```python
from build123d import *

# Parameters (mm, degrees)
SKETCH_1_W          = 8
SKETCH_1_H          = 8
EXTRUDE_1_DEPTH     = 35
SKETCH_2_R          = 1.65
CUT_EXTRUDE_1_DEPTH = 40
SKETCH_3_R          = 1.65
CUT_EXTRUDE_2_DEPTH = 40
SKETCH_6_R          = 1.5
CUT_EXTRUDE_4_DEPTH = 37.783148315
HOLE_WIZARD_M4_3_D  = 3.3


with BuildPart() as part:
    # 草图1 → 凸台-拉伸1 (new body)
    with BuildSketch(Plane.XY):
        with Locations((4, 4)):
            Rectangle(SKETCH_1_W, SKETCH_1_H)
    extrude(amount=EXTRUDE_1_DEPTH)

    # 草图2 → 切除-拉伸1 (cut)
    with BuildSketch(Plane(origin=(8, 0, 0), x_dir=(0, 0, -1), z_dir=(1, 0, 0))):
        with Locations(Location((-32.5, 4, 0), (0, 0, 90))):
            Circle(SKETCH_2_R)
        with Locations(Location((-2.5, 4, 0), (0, 0, 90))):
            Circle(SKETCH_2_R)
    extrude(amount=-CUT_EXTRUDE_1_DEPTH, mode=Mode.SUBTRACT)

    # 草图3 → 切除-拉伸2 (cut)
    with BuildSketch(Plane(origin=(0, 8, 0), x_dir=(1, 0, 0), z_dir=(0, 1, 0))):
        with Locations(Location((4, -17.5, 0), (0, 0, 270))):
            Circle(SKETCH_3_R)
    extrude(amount=-CUT_EXTRUDE_2_DEPTH, mode=Mode.SUBTRACT)

    # 草图6 → 切除-拉伸4 (cut, through all)
    with BuildSketch(Plane(origin=(8, 0, 0), x_dir=(0, 0, -1), z_dir=(1, 0, 0))):
        with Locations(Location((-17.5, 4, 0), (0, 0, 90))):
            Circle(SKETCH_6_R)
    extrude(amount=-CUT_EXTRUDE_4_DEPTH, mode=Mode.SUBTRACT)

    # M4 螺纹孔3 (through all)
    with Locations(Plane(origin=(8, 0, 0), x_dir=(0, 0, -1), z_dir=(1, 0, 0))):
        with Locations((-17.5, 4)):
            Hole(HOLE_WIZARD_M4_3_D / 2)


solid = part.part
```
Input: part model. Units: mm. Frame: model coordinates. Give positions to 0.01 mm unless a question says otherwise; leave off trailing zeros. Order: outer loops, then holes, each group sorted by start corner. A loop starts at its lowest first (then second) coordinate and runs counter-clockwise, first axis right, second up. Notation, with made-up numbers: (72, 11.25) - (120, 11.25) arc R18 ccw to (120, 26.25) - close; hole circle Ø9 at (69, 38.25). An arc over 180 degrees is marked (long way). One line per item, written item: value.
1. Cut plane B-B, the plane z = 32.5. Output: boundary loops of the cut face in (x, y), and give its area (3 significant figures).
Determined:
outline: (0, 0) - (8, 0) - (8, 2.35) - (0, 2.35) - close; (0, 5.65) - (8, 5.65) - (8, 8) - (0, 8) - close
area: 37.6 mm2
2. Line query: probe 1 along Z at (x, y) = (4.5, 4); probe 2 along X at (y, z) = (5.7, 17.5); probe 3 along Z at (x, y) = (2, 5). Output: solid intervals per line, ascending.
Determined:
probe 1: 0 to 0.85, 4.15 to 15.85, 19.15 to 30.85, 34.15 to 35
probe 2: 0 to 2.35, 5.65 to 8
probe 3: 0 to 1.19, 3.81 to 16.19, 18.81 to 31.19, 33.81 to 35
3. Cut plane C-C, the plane y = 6.75. Output: boundary loops of the cut face in (x, z).
Determined:
outline: (0, 0) - (8, 0) - (8, 35) - (0, 35) - close; hole circle Ø3.3 at (4, 17.5)
4. Draft query along Z for faces 1 (the face through (6, 8, 17)), 2 (the face through (1.53, 4.07, 15.85)), 3 (the face through (4, 4, 0)). Return one class per face: released by +Z, released by -Z, zero draft, split by the parting line, or undercut.
Determined:
face 1: zero draft
face 2: undercut
face 3: released by -Z
5. Pin query (flat end, axial travel): pin 1 Ø3 at (y, z) = (4, 17.5) entering from +X. Return the tip coordinate at first contact, or that it passes through.
Determined:
pin 1: through
6. Cut plane D-D, the plane x = 7. Output: boundary loops of the cut face in (y, z), and give its area (3 significant figures).
Determined:
outline: (0, 0) - (8, 0) - (8, 35) - (0, 35) - close; hole circle Ø3.3 at (4, 2.5); hole circle Ø3.3 at (4, 17.5); hole circle Ø3.3 at (4, 32.5)
area: 254 mm2
7. Cut plane A-A, the plane x = 3.25. Output: boundary loops of the cut face in (y, z), and give its area (3 significant figures).
Determined:
outline: (0, 0) - (8, 0) - (8, 16.03) - (4.75, 16.03) arc R1.65 cw to (3.25, 16.03) - (0, 16.03) - close; (0, 18.97) - (3.25, 18.97) arc R1.65 cw to (4.75, 18.97) - (8, 18.97) - (8, 35) - (0, 35) - close; hole circle Ø3.3 at (4, 2.5); hole circle Ø3.3 at (4, 32.5)
area: 239 mm2
